The figure shows three views and two pictorial views of one solid part (mm, origin at its lowest corner). Answer the questions. A direction names the side the tool comes from. Round coordinates to 2 decimals unless told otherwise and drop trailing zeros. Order: outer loops, then holes, each group sorted by start corner. A loop starts at its lowest first (then second) coordinate and runs counter-clockwise, first axis right, second up. Notation, with made-up numbers: (79.25, 33.5) - (97.25, 33.5) arc R33 cw to (97.25, 70.5) - close; hole circle Ø1 at (38, 15). An arc over 180 degrees is marked (long way). One line per item, written item: value. Start each with the question number.
1. Section A-A, the plane x = 31.75 is taken. Give the vertices of the cut face in (y, z).
2. A tool of negligible diameter and unlimited length cuts with its end or side. For the marked faces 4 and 5, from which of +Z, -Z, +X, -X, +Y, -Y can it reach the whole face along a straight path? Write none if from no direction.
3. Section C-C, the plane y = 8.75 is taken. Count the separate pieces of the cut face and the enclosed holes in it, then the cut area to 3 significant figures.
4. Flat-ended cylindrical pins translate along their axes: P1, Ø3, axis at x = 26, y = 9.5, coming from the +Z side; P2, Ø5.5, axis at x = 31.75, z = 9.75, coming from the +Y side; P3, Ø6.5, axis at x = 11, z = 41.5, coming from the -Y side; P4, Ø3, axis at x = 18.5, y = 10.5, coming from the +Z side (1 decimal). Find the tip coordinate at first contact, or state that the pin passes through.
5. Straight lines are drawn through the part: line 1 (Z direction, x = 50.8, y = 2.25); line 2 (Z direction, x = 31.75, y = 9.5); line 3 (Y direction, x = 8, z = 45.5). For each, find the intervals that lie inside material, in ascending order.
6. Section B-B, the plane y = 3.25 is taken. Give the vertices of the cut face in (x, z).
7. For a pull along X with two mould halves and no side action, classify the marked faces 1, 2 and 3 as released by +X, released by -X, zero draft, split by the parting line, or undercut.
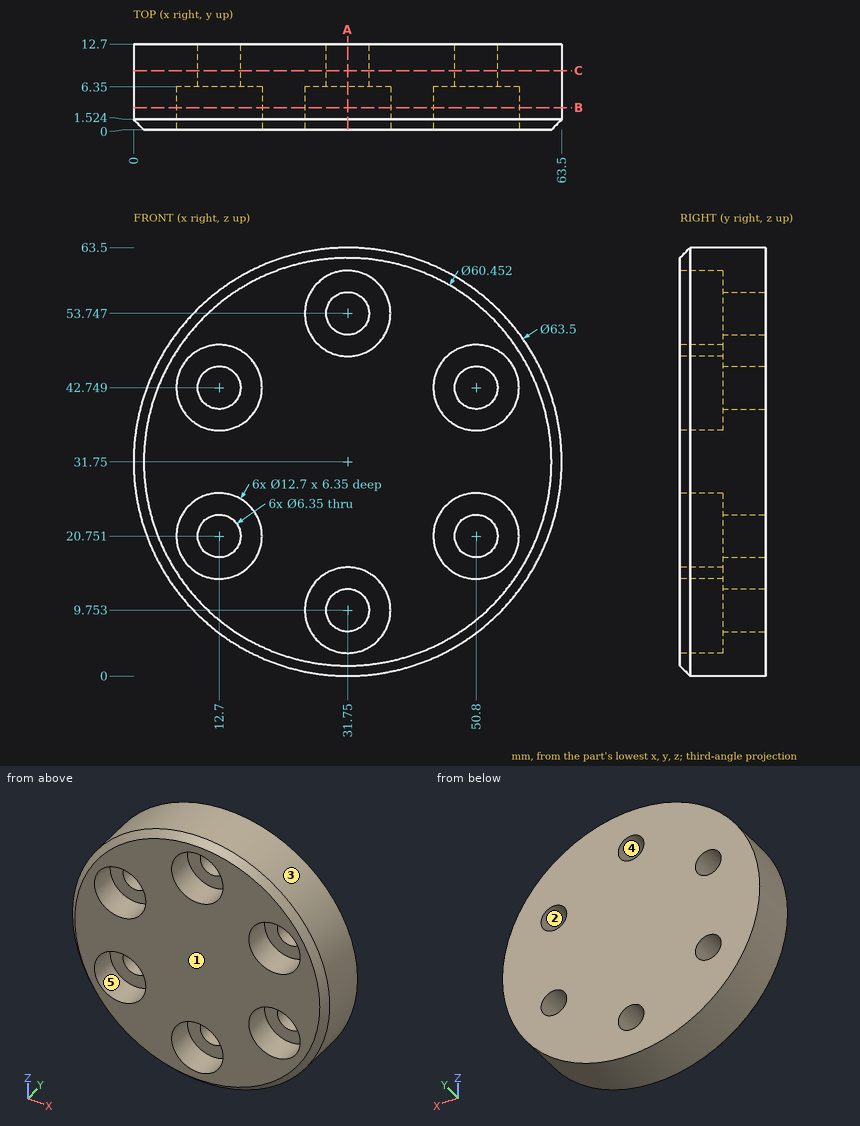
Answer list:
1. outline: (0, 1.52) - (1.52, 0) - (12.7, 0) - (12.7, 6.58) - (6.35, 6.58) - (6.35, 3.4) - (0, 3.4) - close; (0, 16.1) - (6.35, 16.1) - (6.35, 12.93) - (12.7, 12.93) - (12.7, 50.57) - (6.35, 50.57) - (6.35, 47.4) - (0, 47.4) - close; (0, 60.1) - (6.35, 60.1) - (6.35, 56.92) - (12.7, 56.92) - (12.7, 63.5) - (1.52, 63.5) - (0, 61.98) - close
2. face 4: +Y, -Y
2. face 5: -Y
3. separate pieces: 1
3. enclosed holes: 6
3. area: 2,980 mm²
4. P1: stops at z = 63.21
4. P2: passes through
4. P3: stops at y = 6.35
4. P4: stops at z = 61.2
5. line 1: z = 6.35 to 14.4, 27.1 to 36.4, 49.1 to 57.15
5. line 2: z = 0 to 6.58, 12.93 to 50.57, 56.92 to 63.5
5. line 3: y = 6.35 to 12.7
6. outline: circle Ø63.5 at (31.75, 31.75); hole circle Ø12.7 at (12.7, 20.75); hole circle Ø12.7 at (12.7, 42.75); hole circle Ø12.7 at (31.75, 9.75); hole circle Ø12.7 at (31.75, 53.75); hole circle Ø12.7 at (50.8, 20.75); hole circle Ø12.7 at (50.8, 42.75)
7. face 1: zero draft
7. face 2: undercut
7. face 3: split by the parting line
